Can you work these out from the model? Positions are in its coordinate system, mm. Give positions to 0.01 mm unless a question says otherwise; leave off trailing zeros. Order: outer loops, then holes, each group sorted by start corner. A loop starts at its lowest first (then second) coordinate and runs counter-clockwise, first axis right, second up. Notation, with made-up numbers: (-32.5, -4) -> (-4.5, -4) arc R9 cw to (-4.5, 10) -> close; hole circle Ø6 at (31, 42). An arc over 180 degrees is marked (long way). Answer as a JSON object with one key per item and string values.
```python
from build123d import *

# Parameters (mm, degrees)
SKETCH1_R                       = 45
SKETCH1_R_2                     = 1.5
BOSS_EXTRUDE2_DEPTH             = 5
SKETCH9_R                       = 3.937
BOSS_EXTRUDE7_DEPTH             = 4
SKETCH10_R                      = 1.7
CUT_EXTRUDE9_DEPTH              = 14
BOSS_EXTRUDE8_DEPTH             = 5
FILLET1_R                       = 8
SKETCH17_R                      = 8.317724374
BOSS_EXTRUDE9_DEPTH             = 10
CIRPATTERN1_COUNT               = 4
FILLET1_OF_CIRPATTERN1_R        = 8
CUT_EXTRUDE10_DEPTH             = 80.287191735
CUT_EXTRUDE10_DEPTH_BACK        = 80.287191735
SKETCH18_W                      = 16.635448748
SKETCH18_H                      = 10
SKETCH18_W_2                    = 61.874
SKETCH18_H_2                    = 4
M3X0_5_TAPPED_HOLE1_D           = 2.5
M3X0_5_TAPPED_HOLE1_DEPTH       = 3.248924226
M3X0_5_TAPPED_HOLE1_CSINK_D     = 3.05
M3X0_5_TAPPED_HOLE1_CSINK_ANGLE = 90
M3X0_5_TAPPED_HOLE1_TIP         = 0.751075774


with BuildPart() as part:
    # Sketch1 → Boss-Extrude2 (new body)
    with BuildSketch(Plane(origin=(0, 0, 0), x_dir=(1, 0, 0), z_dir=(0, 1, 0))):
        with Locations(Location((0, 0, 0), (0, 0, 270))):
            Circle(SKETCH1_R)
        with Locations(Location((0, 41.75, 0), (0, 0, 270))):
            Circle(SKETCH1_R_2, mode=Mode.SUBTRACT)
        with Locations(Location((29.521708115, 29.521708115, 0), (0, 0, 270))):
            Circle(SKETCH1_R_2, mode=Mode.SUBTRACT)
        with Locations(Location((41.75, 0, 0), (0, 0, 270))):
            Circle(SKETCH1_R_2, mode=Mode.SUBTRACT)
        with Locations(Location((29.521708115, -29.521708115, 0), (0, 0, 270))):
            Circle(SKETCH1_R_2, mode=Mode.SUBTRACT)
        with Locations(Location((0, -41.75, 0), (0, 0, 270))):
            Circle(SKETCH1_R_2, mode=Mode.SUBTRACT)
        with Locations(Location((-29.521708115, -29.521708115, 0), (0, 0, 270))):
            Circle(SKETCH1_R_2, mode=Mode.SUBTRACT)
        with Locations(Location((-41.75, 0, 0), (0, 0, 270))):
            Circle(SKETCH1_R_2, mode=Mode.SUBTRACT)
        with Locations(Location((-29.521708115, 29.521708115, 0), (0, 0, 270))):
            Circle(SKETCH1_R_2, mode=Mode.SUBTRACT)
    extrude(amount=BOSS_EXTRUDE2_DEPTH)

    # Sketch9 → Boss-Extrude7 (add)
    with BuildSketch(Plane.XZ):
        with Locations(Location((27, 0, 0), (0, 0, 90))):
            Circle(SKETCH9_R)
        with Locations(Location((0, -27, 0), (0, 0, 90))):
            Circle(SKETCH9_R)
        with Locations(Location((-27, 0, 0), (0, 0, 90))):
            Circle(SKETCH9_R)
        with Locations(Location((0, 27, 0), (0, 0, 90))):
            Circle(SKETCH9_R)
    extrude(amount=BOSS_EXTRUDE7_DEPTH)

    # Sketch10 → Cut-Extrude9 (cut)
    with BuildSketch(Plane(origin=(0, 5, 0), x_dir=(1, 0, 0), z_dir=(0, 1, 0))):
        with Locations(Location((0, 41.75, 0), (0, 0, 270))):
            Circle(SKETCH10_R)
        with Locations(Location((29.521708115, 29.521708115, 0), (0, 0, 270))):
            Circle(SKETCH10_R)
        with Locations(Location((41.75, 0, 0), (0, 0, 270))):
            Circle(SKETCH10_R)
        with Locations(Location((29.521708115, -29.521708115, 0), (0, 0, 270))):
            Circle(SKETCH10_R)
        with Locations(Location((0, -41.75, 0), (0, 0, 270))):
            Circle(SKETCH10_R)
        with Locations(Location((-29.521708115, -29.521708115, 0), (0, 0, 270))):
            Circle(SKETCH10_R)
        with Locations(Location((-41.75, 0, 0), (0, 0, 270))):
            Circle(SKETCH10_R)
        with Locations(Location((-29.521708115, 29.521708115, 0), (0, 0, 270))):
            Circle(SKETCH10_R)
    extrude(amount=-CUT_EXTRUDE9_DEPTH, mode=Mode.SUBTRACT)

    # Sketch16 → Boss-Extrude8 (add)
    with BuildSketch(Plane.XZ):
        with BuildLine():
            ThreePointArc((45.376634658, -26.343140039), (41.586295626, -22.556734731), (41.583514038, -17.199167429))
            ThreePointArc((41.583514038, -17.199167429), (40.114970744, -20.390907832), (38.401897955, -23.458351039))
            Line((38.401897955, -23.458351039), (45.376634658, -26.343140039))
        make_face()
        with BuildLine():
            Line((50.727486729, -13.406046775), (43.752750026, -10.521257775))
            ThreePointArc((43.752750026, -10.521257775), (42.798576033, -13.902585715), (41.583514038, -17.199167429))
            ThreePointArc((41.583514038, -17.199167429), (45.36991937, -13.408828339), (50.727486729, -13.406046775))
        make_face()
        with BuildLine():
            Line((45.972884991, -19.014635038), (41.583514062, -17.199167371))
            ThreePointArc((41.583514062, -17.199167371), (41.586295614, -22.556734702), (45.376634658, -26.343140039))
            Line((45.376634658, -26.343140039), (47.192102325, -21.95376911))
            ThreePointArc((47.192102325, -21.95376911), (45.973779061, -20.736710252), (45.972884991, -19.014635038))
        make_face()
        with BuildLine():
            ThreePointArc((50.727486729, -13.406046775), (45.369919398, -13.408828327), (41.583514062, -17.199167371))
            Line((41.583514062, -17.199167371), (45.972884991, -19.014635038))
            ThreePointArc((45.972884991, -19.014635038), (47.189943849, -17.796311774), (48.912019062, -17.795417704))
            Line((48.912019062, -17.795417704), (50.727486729, -13.406046775))
        make_face()
        with BuildLine():
            ThreePointArc((55.052060694, -19.874593407), (53.871338237, -15.984091013), (50.727486729, -13.406046775))
            Line((50.727486729, -13.406046775), (48.912019062, -17.795417704))
            ThreePointArc((48.912019062, -17.795417704), (49.922542761, -18.62407478), (50.302060694, -19.874593407))
            ThreePointArc((50.302060694, -19.874593407), (49.30257932, -21.745075474), (47.192102325, -21.95376911))
            Line((47.192102325, -21.95376911), (45.376634658, -26.343140039))
            ThreePointArc((45.376634658, -26.343140039), (51.942563088, -25.69387095), (55.052060694, -19.874593407))
        make_face()
    boss_extrude8 = extrude(amount=-BOSS_EXTRUDE8_DEPTH)

    # Fillet1
    fillet1_edges = [part.edges().sort_by_distance(p)[0] for p in [
        (38.401897955, 2.5, -23.458351039),
        (43.752750026, 2.5, -10.521257775),
    ]]
    fillet(fillet1_edges, radius=FILLET1_R)

    # Sketch17 → Boss-Extrude9 (add)
    with BuildSketch(Plane(origin=(0, 5, 0), x_dir=(1, 0, 0), z_dir=(0, 1, 0))):
        with Locations(Location((0, 0, 0), (0, 0, 270))):
            Circle(SKETCH17_R)
    extrude(amount=BOSS_EXTRUDE9_DEPTH)

    # CirPattern1: Boss-Extrude8 ×4 about axis
    cirpattern1_axis = Axis((0, 0, 0), (0, 1, 0))
    for i in range(1, CIRPATTERN1_COUNT):
        add(boss_extrude8.rotate(cirpattern1_axis, i * 360 / CIRPATTERN1_COUNT))

    # Fillet1 of CirPattern1
    fillet1_of_cirpattern1_edges = [part.edges().sort_by_distance(p)[0] for p in [
        (-23.458351039, 2.5, -38.401897955),
        (-10.521257775, 2.5, -43.752750026),
        (-38.401897955, 2.5, 23.458351039),
        (-43.752750026, 2.5, 10.521257775),
        (23.458351039, 2.5, 38.401897955),
        (10.521257775, 2.5, 43.752750026),
    ]]
    fillet(fillet1_of_cirpattern1_edges, radius=FILLET1_OF_CIRPATTERN1_R)

    # Sketch18 → Cut-Extrude10 (cut, two sides: drawn at the far end of the back side and taken through both)
    with BuildSketch(Plane.XY.offset(-CUT_EXTRUDE10_DEPTH_BACK)):
        with Locations((0, 10)):
            Rectangle(SKETCH18_W, SKETCH18_H)
        with Locations((0, -2)):
            Rectangle(SKETCH18_W_2, SKETCH18_H_2)
    extrude(amount=CUT_EXTRUDE10_DEPTH + CUT_EXTRUDE10_DEPTH_BACK, mode=Mode.SUBTRACT)

    # M3x0.5 Tapped Hole1
    with Locations(Plane(origin=(0, 0, 0), x_dir=(-1, 0, 0), z_dir=(0, -1, 0))):
        with Locations((-18.481561805, 7.644074387), (7.644074387, 18.481561805), (18.481561805, -7.644074387), (-7.644074387, -18.481561805)):
            CounterSinkHole(M3X0_5_TAPPED_HOLE1_D / 2, M3X0_5_TAPPED_HOLE1_CSINK_D / 2, depth=M3X0_5_TAPPED_HOLE1_DEPTH, counter_sink_angle=M3X0_5_TAPPED_HOLE1_CSINK_ANGLE)
            with Locations((0, 0, -(M3X0_5_TAPPED_HOLE1_DEPTH + M3X0_5_TAPPED_HOLE1_TIP / 2))):  # 118° drill point
                Cone(0, M3X0_5_TAPPED_HOLE1_D / 2, M3X0_5_TAPPED_HOLE1_TIP, mode=Mode.SUBTRACT)


solid = part.part
```
1. If we section it at B-B on z = -41.75: Please give me the cut outline in (x, y).
Worked answers:
{"outline": "(-25.31, 0) -> (-1.7, 0) -> (-1.7, 5) -> (-25.31, 5) -> close; (1.7, 0) -> (16.79, 0) -> (16.79, 5) -> (1.7, 5) -> close"}
2. Please list where these lines run through material, in increasing order: L1, parallel to X at y = 2.25, z = 0; L2, parallel to Z at x = 1.5, y = 2.7 (3 decimals); L3, parallel to X at y = 2.35, z = -8.
Worked answers:
{"L1": "-45 to -43.45, -40.05 to 40.05, 43.45 to 45", "L2": "-44.975 to -42.55, -40.95 to 40.95, 42.55 to 44.975", "L3": "-44.28 to 17.28, 19.68 to 45.09"}
3. Will these pins go through, and if not, where does the flat tip stop? pin 1 Ø3 at (x, z) = (41.75, 0) entering from +Y; pin 2 Ø1.5 at (x, z) = (-7.64, -18.48) entering from -Y; pin 3 Ø2 at (x, z) = (18.48, -7.64) entering from -Y.
Worked answers:
{"pin 1": "through", "pin 2": "y = 3.55", "pin 3": "y = 3.4"}
4. If we section it at D-D on y = 2.1: Count the separate pieces of the cut face and the enclosed holes in it, then the cut area to 3 significant figures.
Worked answers:
{"separate pieces": "1", "enclosed holes": "16", "area": "6,980 mm²"}
5. If we mould it in two halves opening along X, with no side actions, what happens to faces 1 (the face through (39.194, 2.535, -25.556)), 2 (the face through (1, 5, -1)), 3 (the face through (-25.52, 2.54, -39.33))? For each: +X half, -X half, draft (parallel to the pull), parting line (faces both ways), or undercut.
Worked answers:
{"face 1": "undercut", "face 2": "draft", "face 3": "-X half"}
6. If we section it at C-C on x = 41.75: Please give me the cut outline in (y, z), then the cut area to 3 significant figures.
Worked answers:
{"outline": "(0, -25.31) -> (5, -25.31) -> (5, -1.7) -> (0, -1.7) -> close; (0, 1.7) -> (5, 1.7) -> (5, 16.79) -> (0, 16.79) -> close", "area": "193 mm²"}
7. If we section it at A-A on x = 0: Please give me the cut outline in (y, z), then the cut area to 3 significant figures.
Worked answers:
{"outline": "(0, -45) -> (5, -45) -> (5, -43.45) -> (0, -43.45) -> close; (0, -40.05) -> (5, -40.05) -> (5, 40.05) -> (0, 40.05) -> close; (0, 43.45) -> (5, 43.45) -> (5, 45) -> (0, 45) -> close", "area": "416 mm²"}
